Autodesk Inventor part; units mm, degrees
ref_plane "YZ Plane" through (0, 0, 0) normal (1, 0, 0) x (0, 1, 0)
ref_plane "XZ Plane" through (0, 0, 0) normal (0, 1, 0) x (-1, 0, 0)
ref_plane "XY Plane" through (0, 0, 0) normal (0, 0, 1) x (1, 0, 0)
sketch "Sketch1" plane through (0, 0, 0) normal (0, 1, 0) x (-1, 0, 0)
  line L0 (0, 0) -> (-24, 0)
  line L1 (-24, 0) -> (-24, 44)
  line L2 (-24, 44) -> (0, 44)
  line L3 (0, 44) -> (0, 0)
  dimension "d0" = 24
  dimension "d1" = 44
extrude "Extrusion1" add sketch "Sketch1" along normal blind 1.6
sketch "Sketch3" plane through (0, 1.6, 0) normal (0, 1, 0) x (1, 0, 0)
  line L0 (3.6828, -4.4062) -> (20.3867, -4.4062)
  line L1 (20.3867, -4.4062) -> (20.3867, -35.052)
  line L2 (20.3867, -35.052) -> (3.6828, -35.052)
  line L3 (3.6828, -35.052) -> (3.6828, -4.4062)
  line L4 (4.8665, -37.9456) -> (18.6769, -37.9456)
  line L5 (18.6769, -37.9456) -> (18.6769, -41.7599)
  line L6 (18.6769, -41.7599) -> (4.8665, -41.7599)
  line L7 (4.8665, -41.7599) -> (4.8665, -37.9456)
  point P0 (0, 0)
extrude "Extrusion3" add sketch "Sketch3" along normal blind 1.6 contours L0 L1 L2 L3
sketch "Sketch4" plane through (0, 1.6, 0) normal (0, 1, 0) x (1, 0, 0)
  point P0 (0, 0)
properties part number "Gyro"
Geometry check sheet. Reference: the model listing, model coordinates, mm. A direction names the side the tool comes from. Round coordinates to 2 decimals unless told otherwise and drop trailing zeros. Loops run counter-clockwise (first coordinate to the right, second up) from the corner with the lowest first, then second, coordinate; pieces in that order, holes last.
Item 1: Cross-section at B-B on z = 27. Record the boundary of the cut face in (x, y).
Item 2: Gauge pin test, flat ends, axial feed: pin 1 (1 mm diameter, centred on x = 18, z = 39.5, fed in from +Y); pin 2 (1 mm diameter, centred on y = 1, z = 35.5, fed in from -X); pin 3 (0.8 mm diameter, centred on y = 2.5, z = 25.5, fed in from -X); pin 4 (1.3 mm diameter, centred on x = 16, y = 2.5, fed in from +Z). Record the tip position at first contact, or that the pin passes through.
Item 3: Cross-section at A-A on x = 15. Record the boundary of the cut face in (y, z), then the cut area to 3 significant figures.
Item 4: Thickness scan on line 1 (Z direction, x = 3.75, y = 2.7); line 2 (X direction, y = 1.95, z = 5); line 3 (Y direction, x = 5.5, z = 3). Record the ranges inside material, lowest first.
Item 5: Cross-section at D-D on z = 37. Record the boundary of the cut face in (x, y).
Item 6: Access from +Z, -Z, +X, -X, +Y, -Y to the whole of each face (thin tool, end or side, straight path). Record for faces 1 (the flat face through (12, 2, 35.052)), 2 (the flat face through (20.387, 2, 20)), 3 (the flat face through (3.683, 2, 20)), 4 (the flat face through (12, 2, 4.406)).
Item 7: Cross-section at C-C on y = 2.5. Record the boundary of the cut face in (x, z), then the cut area to 3 significant figures.
Answer sheet:
1. outline: (0, 0) - (24, 0) - (24, 1.6) - (20.39, 1.6) - (20.39, 3.2) - (3.68, 3.2) - (3.68, 1.6) - (0, 1.6) - close
2. pin 1: stops at y = 1.6
2. pin 2: stops at x = 0
2. pin 3: stops at x = 3.68
2. pin 4: stops at z = 35.05
3. outline: (0, 0) - (1.6, 0) - (1.6, 4.41) - (3.2, 4.41) - (3.2, 35.05) - (1.6, 35.05) - (1.6, 44) - (0, 44) - close
3. area: 119 mm2
4. line 1: z = 4.41 to 35.05
4. line 2: x = 3.68 to 20.39
4. line 3: y = 0 to 1.6
5. outline: (0, 0) - (24, 0) - (24, 1.6) - (0, 1.6) - close
6. face 1: +Z, +X, -X, +Y
6. face 2: +Z, -Z, +X, +Y
6. face 3: +Z, -Z, -X, +Y
6. face 4: -Z, +X, -X, +Y
7. outline: (3.68, 4.41) - (20.39, 4.41) - (20.39, 35.05) - (3.68, 35.05) - close
7. area: 512 mm2
